Input: part model. Units: mm. Frame: model coordinates. Face numbers are marked on the shaded views. A direction names the side the tool comes from. Coordinates: 2 decimals unless noted, no trailing zeros. Loops run counter-clockwise (first coordinate to the right, second up) from the corner with the lowest first, then second, coordinate; pieces in that order, holes last. Notation, with made-up numbers: (51, -0.75) -> (85, -0.75) arc R23 cw to (85, 25.25) -> close; hole circle Ø3 at (4.25, 25.25). An arc over 180 degrees is marked (long way). Answer as a JSON object with one key per item and string values.
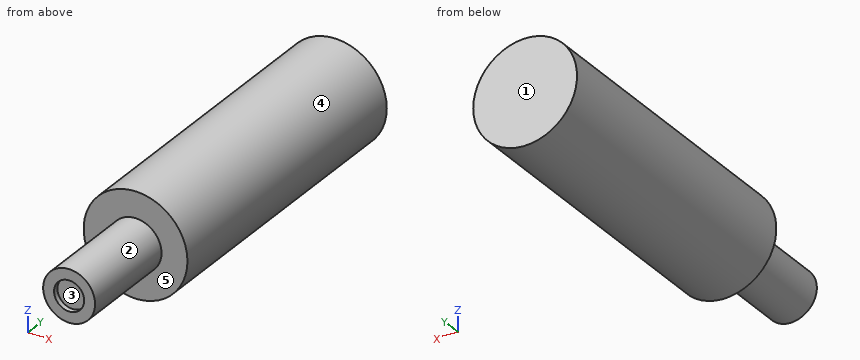
from build123d import *

# Parameters (mm, degrees)
F0_R     = 5
F1_DEPTH = 40
F2_R     = 5.5
F2_R_2   = 2.5
F3_DEPTH = 10
F4_R     = 1.45
F5_DEPTH = 0.5


with BuildPart() as f1:
    # F0 (on Front) → F1 (new body)
    with BuildSketch(Plane.XZ):
        Circle(F0_R)
    extrude(amount=F1_DEPTH)

    # F2 (on face) → F3 (cut)
    with BuildSketch(Plane.XZ.offset(40)):
        Circle(F2_R)
        Circle(F2_R_2, mode=Mode.SUBTRACT)
    extrude(amount=-F3_DEPTH, mode=Mode.SUBTRACT)

    # F4 (on face) → F5 (cut)
    with BuildSketch(Plane.XZ.offset(40)):
        Circle(F4_R)
    extrude(amount=-F5_DEPTH, mode=Mode.SUBTRACT)


solid = f1.part
1. Section query D-D (y = -8.5). Return loops of the section in (x, z), plus the area to 3 significant figures.
Reply:
{"outline": "circle Ø10 at (0, 0)", "area": "78.5 mm2"}
2. Mould query, pull axis Z, two halves, no side actions, for the marked faces 1, 2 and 3. Classes: pulls with the +Z half, pulls with the -Z half, needs draft (parallel to the pull), parting line crosses it, or undercut.
Reply:
{"face 1": "needs draft", "face 2": "parting line crosses it", "face 3": "undercut"}
3. Section query B-B (z = 0). Return loops of the section in (x, y).
Reply:
{"outline": "(-5, -30) -> (-2.5, -30) -> (-2.5, -40) -> (-1.45, -40) -> (-1.45, -39.5) -> (1.45, -39.5) -> (1.45, -40) -> (2.5, -40) -> (2.5, -30) -> (5, -30) -> (5, 0) -> (-5, 0) -> close"}
4. Section query C-C (y = -31.5). Return loops of the section in (x, z).
Reply:
{"outline": "circle Ø5 at (0, 0)"}
5. Section query A-A (x = 0). Return loops of the section in (y, z), plus the area to 3 significant figures.
Reply:
{"outline": "(-40, -2.5) -> (-30, -2.5) -> (-30, -5) -> (0, -5) -> (0, 5) -> (-30, 5) -> (-30, 2.5) -> (-40, 2.5) -> (-40, 1.45) -> (-39.5, 1.45) -> (-39.5, -1.45) -> (-40, -1.45) -> close", "area": "349 mm2"}
6. Access query for the marked faces 4 and 5. Directions: +Z, -Z, +X, -X, +Y, -Y. A direction counts if a zero-diameter tool reaches every point of the face in a straight line with its end or side. Return the directions, or none.
Reply:
{"face 4": "+Y, -Y", "face 5": "-Y"}
7. Line query: line 1 along Z through (x, y) = (0, -39.8); line 2 along Y through (x, z) = (3.5, 2.75); line 3 along Y through (x, z) = (0.5, 0). Output: solid intervals per line, ascending.
Reply:
{"line 1": "z = -2.5 to -1.45, 1.45 to 2.5", "line 2": "y = -30 to 0", "line 3": "y = -39.5 to 0"}
8. Pin query (flat end, axial travel): P1, Ø2, axis at y = -26, z = -3.5, coming from the +X side; P2, Ø2, axis at x = 1.5, z = -2.5, coming from the +Y side; P3, Ø1.4, axis at x = 0.5, z = -0.5, coming from the -Y side; P4, Ø1, axis at x = 3.5, y = -16.5, coming from the +Z side. Return the tip coordinate at first contact, or that it passes through.
Reply:
{"P1": "stops at x = 4.33", "P2": "stops at y = 0", "P3": "stops at y = -39.5", "P4": "stops at z = 4"}
